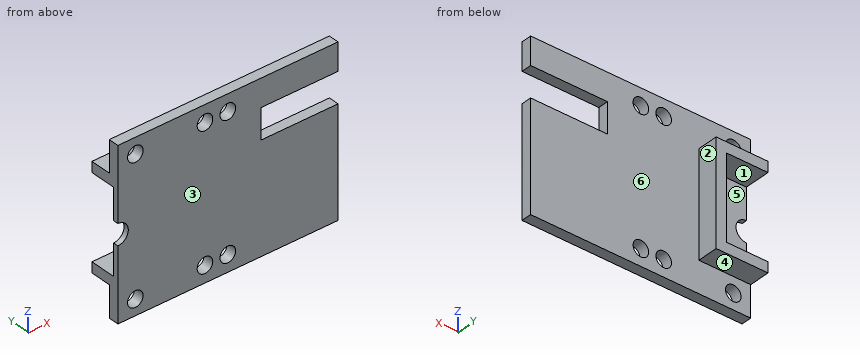
from build123d import *

# Parameters (mm, degrees)
SKETCH1_W                = 279.4
SKETCH1_H                = 101.6
BOSS_EXTRUDE1_DEPTH      = 6.35
SKETCH2_R                = 13.97
BOSS_EXTRUDE3_DEPTH      = 5.55625
SKETCH9_R                = 11.1125
CUT_EXTRUDE4_DEPTH       = 4.445
CUT_EXTRUDE5_START       = -5.55625
SKETCH10_R               = 11.1125
CUT_EXTRUDE5_DEPTH       = 5.55625
SKETCH11_R               = 7.9375
CUT_EXTRUDE6_DEPTH       = 285.078633923
SKETCH12_R               = 6.35
CUT_EXTRUDE7_DEPTH       = 285.051619429
SKETCH22_W               = 63.5
SKETCH22_H               = 63.5
BOSS_EXTRUDE7_DEPTH      = 12.7
SKETCH25_W               = 50.8
SKETCH25_H               = 50.8
CUT_EXTRUDE11_DEPTH      = 15.875
SKETCH32_R               = 4.7625
CUT_EXTRUDE12_DEPTH      = 6.35
SKETCH38_W               = 46.99
SKETCH38_H               = 18.470251096
CUT_EXTRUDE13_DEPTH      = 6.35
SKETCH60_R               = 4.7625
CUT_EXTRUDE23_DEPTH      = 6.35
CUT_EXTRUDE26_DEPTH      = 285.264471927
CUT_EXTRUDE26_DEPTH_BACK = 285.264471927
SKETCH63_R               = 4.7625
CUT_EXTRUDE27_DEPTH      = 145.488464724


with BuildPart() as part:
    # Sketch1 → Boss-Extrude1 (new body)
    with BuildSketch(Plane(origin=(0, 0, 0), x_dir=(1, 0, 0), z_dir=(0, 1, 0))):
        with Locations((-139.7, 0)):
            Rectangle(SKETCH1_W, SKETCH1_H)
    extrude(amount=BOSS_EXTRUDE1_DEPTH)

    # Sketch2 → Boss-Extrude3 (add)
    with BuildSketch(Plane(origin=(0, 6.35, 0), x_dir=(1, 0, 0), z_dir=(0, 1, 0))):
        with Locations(Location((-258.510557857, 0, 0), (0, 0, 90))):
            Circle(SKETCH2_R)
    extrude(amount=BOSS_EXTRUDE3_DEPTH)

    # Sketch9 → Cut-Extrude4 (cut)
    with BuildSketch(Plane(origin=(0, 11.90625, 0), x_dir=(1, 0, 0), z_dir=(0, 1, 0))):
        with Locations(Location((-258.510557857, 0, 0), (0, 0, 270))):
            Circle(SKETCH9_R)
    extrude(amount=-CUT_EXTRUDE4_DEPTH, mode=Mode.SUBTRACT)

    # Sketch10 → Cut-Extrude5 (cut)
    with BuildSketch(Plane(origin=(0, 0, 0), x_dir=(-1, 0, 0), z_dir=(0, -1, 0)).offset(CUT_EXTRUDE5_START)):
        with Locations(Location((258.510557857, 0, 0), (0, 0, 270))):
            Circle(SKETCH10_R)
    extrude(amount=CUT_EXTRUDE5_DEPTH, mode=Mode.SUBTRACT)

    # Sketch11 → Cut-Extrude6 (cut, through all)
    with BuildSketch(Plane(origin=(0, 7.46125, 0), x_dir=(1, 0, 0), z_dir=(0, 1, 0))):
        with Locations(Location((-258.510557857, 0, 0), (0, 0, 270))):
            Circle(SKETCH11_R)
    extrude(amount=-CUT_EXTRUDE6_DEPTH, mode=Mode.SUBTRACT)

    # Sketch12 → Cut-Extrude7 (cut, through all)
    with BuildSketch(Plane(origin=(0, 6.35, 0), x_dir=(1, 0, 0), z_dir=(0, 1, 0))):
        with Locations(Location((-134.666203771, 0, 0), (0, 0, 270))):
            Circle(SKETCH12_R)
    extrude(amount=-CUT_EXTRUDE7_DEPTH, mode=Mode.SUBTRACT)

    # Sketch22 → Boss-Extrude7 (add)
    with BuildSketch(Plane(origin=(0, 6.35, 0), x_dir=(1, 0, 0), z_dir=(0, 1, 0))):
        with Locations((-134.666203771, 0)):
            Rectangle(SKETCH22_W, SKETCH22_H)
    extrude(amount=BOSS_EXTRUDE7_DEPTH)

    # Sketch25 → Cut-Extrude11 (cut)
    with BuildSketch(Plane(origin=(0, 19.05, 0), x_dir=(1, 0, 0), z_dir=(0, 1, 0))):
        with Locations((-134.666203771, 0)):
            Rectangle(SKETCH25_W, SKETCH25_H)
    extrude(amount=-CUT_EXTRUDE11_DEPTH, mode=Mode.SUBTRACT)

    # Sketch32 → Cut-Extrude12 (cut)
    with BuildSketch(Plane(origin=(0, 6.35, 0), x_dir=(1, 0, 0), z_dir=(0, 1, 0))):
        with Locations(Location((-67.44195898, -40.64, 0), (0, 0, 270))):
            Circle(SKETCH32_R)
        with Locations(Location((-81.41195898, -40.64, 0), (0, 0, 270))):
            Circle(SKETCH32_R)
        with Locations(Location((-67.44195898, 40.64, 0), (0, 0, 270))):
            Circle(SKETCH32_R)
        with Locations(Location((-81.41195898, 40.64, 0), (0, 0, 270))):
            Circle(SKETCH32_R)
    extrude(amount=-CUT_EXTRUDE12_DEPTH, mode=Mode.SUBTRACT)

    # Sketch38 → Cut-Extrude13 (cut)
    with BuildSketch(Plane(origin=(0, 6.35, 0), x_dir=(1, 0, 0), z_dir=(0, 1, 0))):
        with Locations((-23.495, -24.777709652)):
            Rectangle(SKETCH38_W, SKETCH38_H)
    extrude(amount=-CUT_EXTRUDE13_DEPTH, mode=Mode.SUBTRACT)

    # Sketch60 → Cut-Extrude23 (cut)
    with BuildSketch(Plane(origin=(0, 6.35, 0), x_dir=(1, 0, 0), z_dir=(0, 1, 0))):
        with Locations(Location((-231.7492444, 41.324145444, 0), (0, 0, 270))):
            Circle(SKETCH60_R)
        with Locations(Location((-231.7492444, -39.369341378, 0), (0, 0, 270))):
            Circle(SKETCH60_R)
        with Locations(Location((-173.509244294, -39.369341378, 0), (0, 0, 270))):
            Circle(SKETCH60_R)
        with Locations(Location((-173.509244294, 41.324145444, 0), (0, 0, 270))):
            Circle(SKETCH60_R)
    extrude(amount=-CUT_EXTRUDE23_DEPTH, mode=Mode.SUBTRACT)

    # Sketch62 → Cut-Extrude26 (cut, two sides: drawn at the far end of the back side and taken through both)
    with BuildSketch(Plane(origin=(0, 6.35, 0), x_dir=(1, 0, 0), z_dir=(0, 1, 0)).offset(-CUT_EXTRUDE26_DEPTH_BACK)):
        Polygon((-134.666203771, -414.468951257), (-134.666203771, -50.8), (-134.666203771, 0), (-134.666203771, 50.8), (-134.666203771, 414.468951257), (-862.004106285, 414.468951257), (-862.004106285, -414.468951257), align=None)
    extrude(amount=CUT_EXTRUDE26_DEPTH + CUT_EXTRUDE26_DEPTH_BACK, mode=Mode.SUBTRACT)

    # Sketch63 → Cut-Extrude27 (cut, through all)
    with BuildSketch(Plane(origin=(0, 6.35, 0), x_dir=(1, 0, 0), z_dir=(0, 1, 0))):
        with Locations(Location((-123.998203771, 41.275, 0), (0, 0, 270))):
            Circle(SKETCH63_R)
    cut_extrude27 = extrude(amount=-CUT_EXTRUDE27_DEPTH, mode=Mode.SUBTRACT)

    # Mirror1: Cut-Extrude27 across plane
    add(cut_extrude27.mirror(Plane.XY), mode=Mode.SUBTRACT)


solid = part.part
Read the model definition and answer for the solid it produces. Units are mm, in the model's axes. Face numbers are marked on the shaded views. A direction names the side the tool comes from. Round coordinates to 2 decimals unless told otherwise and drop trailing zeros. Write each loop counter-clockwise with the first axis right and the second up, starting at its lowest first coordinate (ties: lowest second). Pieces come first, ordered by that corner, then holes. Notation, with made-up numbers: (5.5, -30.75) - (48.5, -30.75) arc R30 ccw to (48.5, -2.75) - close; hole circle Ø8 at (-30.75, 42.25). An arc over 180 degrees is marked (long way). Use a Markdown table: item, result.
(1) The mould has two halves that part along Z. Classify the marked faces 4, 5 and 6: released by +Z, released by -Z, zero draft, split by the parting line, or undercut.
Reported:
| item | result |
|---|---|
| face 4 | released by -Z |
| face 5 | undercut |
| face 6 | zero draft |
(2) The part is cut by section B-B (z = 40.64). Write down the section's boundary in (x, y).
Reported:
| item | result |
|---|---|
| outline | (-134.67, 0) - (-128.72, 0) - (-128.72, 6.35) - (-134.67, 6.35) - close; (-119.28, 0) - (-86.17, 0) - (-86.17, 6.35) - (-119.28, 6.35) - close; (-76.65, 0) - (-72.2, 0) - (-72.2, 6.35) - (-76.65, 6.35) - close; (-62.68, 0) - (0, 0) - (0, 6.35) - (-62.68, 6.35) - close |
(3) Which of the six approach directions +Z, -Z, +X, -X, +Y, -Y give full straight-line access (tool end or side, diameter ignored) to the marked faces 1, 2 and 3?
Reported:
| item | result |
|---|---|
| face 1 | -X, +Y |
| face 2 | +Z, -Z, +X, +Y |
| face 3 | +Z, -Z, +X, -X, -Y |
(4) Straight lines are drawn through the part: line 1 along Z through (x, y) = (-125, 7); line 2 along X through (y, z) = (5.25, -40.64); line 3 along Z through (x, y) = (-46, 4). For each, find the intervals that lie inside material, in ascending order. Write a range as [from, to].
Reported:
| item | result |
|---|---|
| line 1 | [-31.75, -25.4], [25.4, 31.75] |
| line 2 | [-134.67, -128.72], [-119.28, -86.17], [-76.65, -72.2], [-62.68, 0] |
| line 3 | [-50.8, 15.54], [34.01, 50.8] |
(5) The part is cut by section D-D (z = 0). Write down the section's boundary in (x, y) (3 decimals).
Reported:
| item | result |
|---|---|
| outline | (-128.316, 0) - (0, 0) - (0, 6.35) - (-102.916, 6.35) - (-102.916, 19.05) - (-109.266, 19.05) - (-109.266, 3.175) - (-128.316, 3.175) - close |
(6) The part is cut by section C-C (y = 14.5). Write down the section's boundary in (x, z).
Reported:
| item | result |
|---|---|
| outline | (-134.67, -31.75) - (-102.92, -31.75) - (-102.92, 31.75) - (-134.67, 31.75) - (-134.67, 25.4) - (-109.27, 25.4) - (-109.27, -25.4) - (-134.67, -25.4) - close |
(7) The part is cut by section A-A (x = -30). Write down the section's boundary in (y, z), then the cut area to 3 significant figures.
Reported:
| item | result |
|---|---|
| outline | (0, -50.8) - (6.35, -50.8) - (6.35, 15.54) - (0, 15.54) - close; (0, 34.01) - (6.35, 34.01) - (6.35, 50.8) - (0, 50.8) - close |
| area | 528 mm2 |
(8) Each of these flat-tipped pins is pushed along its axis until it touches: pin 1 Ø3 at (y, z) = (2, 22) entering from +X; pin 2 Ø8 at (x, y) = (-127.5, 14.5) entering from -Z; pin 3 Ø5 at (y, z) = (7.5, 0.5) entering from -X; pin 4 Ø8.5 at (x, z) = (-67.44, 40.64) entering from -Y. Where does it stop, or does it pass through?
Reported:
| item | result |
|---|---|
| pin 1 | x = -46.99 |
| pin 2 | z = -31.75 |
| pin 3 | x = -109.27 |
| pin 4 | through |
